Print and shaded views of the part. All mm, measured from the part's lowest x, y and z. A direction names the side the tool comes from. Coordinates: 2 decimals unless noted, no trailing zeros. Loops run counter-clockwise (first coordinate to the right, second up) from the corner with the lowest first, then second, coordinate; pieces in that order, holes last. Notation, with made-up numbers: (6.5, 29.25) -> (60.5, 29.25) arc R16 ccw to (60.5, 34.25) -> close; hole circle Ø9 at (47.25, -39). An arc over 180 degrees is marked (long way). One line per item, written item: value. Start each with the question number.
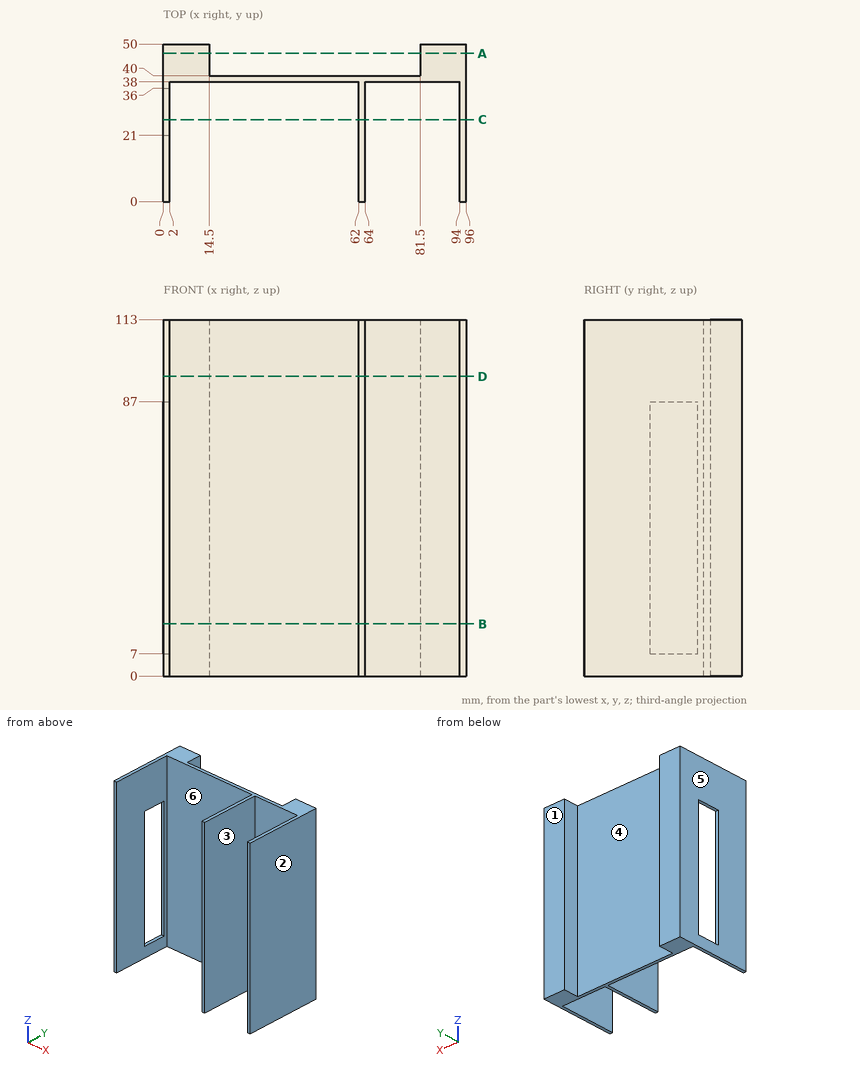
1) Slice it at C-C (y = 26). Give the cut face in (x, z).
2) Tool access for the marked faces 4, 5 and 6: list every direction of +Z, -Z, +X, -X, +Y, -Y with a clear straight run to the whole face (end or side of a thin tool).
3) Slice it at A-A (y = 47). Give the cut face in (x, z).
4) Probe line 1 (X direction, y = 28, z = 104); line 2 (X direction, y = 26.5, z = 54.5); line 3 (X direction, y = 40.5, z = 94). List the from-to ranges inside material, lowest first. Write a range as from..to.
5) Pull direction X, two halves, no side cores. Call the marked faces 1, 2 and 3: +X half, -X half, draft (parallel to the pull), parting line (faces both ways), or undercut.
6) Slice it at D-D (z = 95). Give the cut face in (x, y).
7) Slice it at B-B (z = 16.5). Give the cut face in (x, y), then the cut area to 3 significant figures.
8) Pin check, flat tips, straight feed: pin 1 Ø3 at (x, y) = (68, 37) entering from +Z; pin 2 Ø12 at (x, z) = (70, 17.5) entering from +Y; pin 3 Ø1 at (y, z) = (23, 44.5) entering from -X; pin 4 Ø9 at (x, z) = (85, 55.5) entering from -Y. Stop position of each tip, or through.
Check sheet entries:
1. outline: (0, 0) -> (2, 0) -> (2, 7) -> (0, 7) -> close; (0, 87) -> (2, 87) -> (2, 113) -> (0, 113) -> close; (62, 0) -> (64, 0) -> (64, 113) -> (62, 113) -> close; (94, 0) -> (96, 0) -> (96, 113) -> (94, 113) -> close
2. face 4: +Z, -Z, +Y
2. face 5: +Z, -Z, -X, +Y, -Y
2. face 6: +Z, -Z, -Y
3. outline: (0, 0) -> (14.5, 0) -> (14.5, 113) -> (0, 113) -> close; (81.5, 0) -> (96, 0) -> (96, 113) -> (81.5, 113) -> close
4. line 1: x = 0..2, 62..64, 94..96
4. line 2: x = 62..64, 94..96
4. line 3: x = 0..14.5, 81.5..96
5. face 1: draft
5. face 2: +X half
5. face 3: undercut
6. outline: (0, 0) -> (2, 0) -> (2, 38) -> (62, 38) -> (62, 0) -> (64, 0) -> (64, 38) -> (94, 38) -> (94, 0) -> (96, 0) -> (96, 50) -> (81.5, 50) -> (81.5, 40) -> (14.5, 40) -> (14.5, 50) -> (0, 50) -> close
7. outline: (0, 0) -> (2, 0) -> (2, 21) -> (0, 21) -> close; (0, 36) -> (2, 36) -> (2, 38) -> (62, 38) -> (62, 0) -> (64, 0) -> (64, 38) -> (94, 38) -> (94, 0) -> (96, 0) -> (96, 50) -> (81.5, 50) -> (81.5, 40) -> (14.5, 40) -> (14.5, 50) -> (0, 50) -> close
7. area: 680 mm^2
8. pin 1: stops at z = 113
8. pin 2: stops at y = 40
8. pin 3: stops at x = 62
8. pin 4: stops at y = 38
